Autodesk Inventor part; units mm, degrees
ref_plane "YZ Plane" through (0, 0, 0) normal (1, 0, 0) x (0, 1, 0)
ref_plane "XZ Plane" through (0, 0, 0) normal (0, 1, 0) x (-1, 0, 0)
ref_plane "XY Plane" through (0, 0, 0) normal (0, 0, 1) x (1, 0, 0)
sketch "Náčrt1" plane through (0, 0, 0) normal (0, 0, 1) x (1, 0, 0)
  line L0 (0, 0) -> (-28.2, 0)
  line L1 (-28.2, 0) -> (-28.2, -28.2)
  line L2 (-28.2, -28.2) -> (0, -28.2)
  line L3 (0, -28.2) -> (28.2, -28.2)
  line L4 (28.2, -28.2) -> (28.2, 28.2)
  line L5 (28.2, 28.2) -> (-28.2, 28.2)
  line L6 (-28.2, 28.2) -> (-28.2, 0)
  dimension "d0" = 28.2
  dimension "d1" = 28.2
  dimension "d2" = 28.2
  dimension "d3" = 56.4
extrude "Vysunutí1" add sketch "Náčrt1" along normal blind 54
sketch "Náčrt2" plane through (0, 0, 0) normal (0, 0, -1) x (-1, 0, 0)
  line L0 (28.2, 28.2) -> (28.2, -28.2)
  line L1 (-28.2, 28.2) -> (28.2, 28.2)
  line L2 (-28.2, -28.2) -> (-28.2, 28.2)
  line L3 (28.2, -28.2) -> (-28.2, -28.2)
  line L4 (28.2, 0) -> (28.2, -17.25)
  line L5 (17.25, -28.2) -> (-17.25, -28.2)
  line L6 (-17.25, -28.2) -> (-28.2, -17.25)
  line L7 (-28.2, -17.25) -> (-28.2, 17.25)
  line L8 (-28.2, 17.25) -> (-17.25, 28.2)
  line L9 (17.25, 28.2) -> (28.2, 17.25)
  line L10 (28.2, 17.25) -> (28.2, 0)
  line L11 (28.2, -28.2) -> (19.7, -28.2)
  line L12 (19.7, -28.2) -> (19.7, -19.7)
  line L13 (19.7, -19.7) -> (28.2, -19.7)
  line L14 (28.2, -19.7) -> (28.2, -28.2)
  line L15 (-28.2, -28.2) -> (-19.7, -28.2)
  line L16 (-19.7, -28.2) -> (-19.7, -19.7)
  line L17 (-19.7, -19.7) -> (-28.2, -19.7)
  line L18 (-28.2, -19.7) -> (-28.2, -28.2)
  line L19 (-28.2, 28.2) -> (-19.7, 28.2)
  line L20 (-19.7, 28.2) -> (-19.7, 19.7)
  line L21 (-19.7, 19.7) -> (-28.2, 19.7)
  line L22 (-28.2, 19.7) -> (-28.2, 28.2)
  line L23 (28.2, 28.2) -> (19.7, 28.2)
  line L24 (19.7, 28.2) -> (19.7, 19.7)
  line L25 (19.7, 19.7) -> (28.2, 19.7)
  line L26 (28.2, 19.7) -> (28.2, 28.2)
  line L27 (28.2, 17.25) -> (19.7, 19.7)
  line L28 (17.25, 28.2) -> (19.7, 19.7)
  line L29 (-17.25, 28.2) -> (-19.7, 19.7)
  line L30 (-28.2, 17.25) -> (-19.7, 19.7)
  line L31 (-28.2, -17.25) -> (-19.7, -19.7)
  line L32 (-19.7, -19.7) -> (-17.25, -28.2)
  line L33 (17.25, -28.2) -> (19.7, -19.7)
  line L34 (19.7, -19.7) -> (28.2, -17.25)
  line L35 (28.2, -17.25) -> (25.75, -19.7)
  line L36 (19.7, -25.75) -> (17.25, -28.2)
  point P0 (0, 0)
  dimension "d6" = 17.25
  dimension "d8" = 34.5
  dimension "d9" = 34.5
  dimension "d10" = 8.5
  dimension "d11" = 8.5
  dimension "d12" = 8.5
  dimension "d13" = 8.5
  dimension "d14" = 8.5
extrude "Vysunutí2" add sketch "Náčrt2" along normal blind 49 contours L0 L34 L33 L3 L32 L31 L2 L30 L29 L1 L28 L27
sketch "Náčrt3" plane through (0, 0, 54) normal (0, 0, 1) x (1, 0, 0)
  line L0 (-28.2, -28.2) -> (-28.2, 28.2)
  line L1 (28.2, -28.2) -> (-28.2, -28.2)
  line L2 (28.2, -28.2) -> (-28.2, -28.2)
  line L3 (-28.2, -28.2) -> (-28.2, 28.2)
  line L4 (-28.2, 28.2) -> (28.2, 28.2)
  line L5 (28.2, 28.2) -> (28.2, -28.2)
  point P0 (0, 0)
extrude "Vysunutí3" cut sketch "Náčrt3" against normal blind 49
fillet "Zaoblení1" radius 3 12 edges at (-17.25, -28.2, -24.5) (-19.7, -19.7, -24.5) (-28.2, -17.25, -24.5) (17.25, -28.2, -24.5) (19.7, -19.7, -24.5) (28.2, -17.25, -24.5) (28.2, 17.25, -24.5) (19.7, 19.7, -24.5) (17.25, 28.2, -24.5) (-17.25, 28.2, -24.5) (-19.7, 19.7, -24.5) (-28.2, 17.25, -24.5)
fillet "Zaoblení2" radius 4.6 4 edges at (28.2, 28.2, 2.5) (28.2, -28.2, 2.5) (-28.2, -28.2, 2.5) (-28.2, 28.2, 2.5)
sketch "Náčrt4" plane through (0, 0, 5) normal (0, 0, 1) x (1, 0, 0)
  circle A0 centre (0, 0) radius 19.05
  dimension "d21" = 38.1
extrude "Vysunutí4" add sketch "Náčrt4" along normal blind 1.6
sketch "Náčrt5" plane through (0, 0, 6.6) normal (0, 0, 1) x (1, 0, 0)
  circle A0 centre (0, 0) radius 19.05
  circle A1 centre (0, 0) radius 3.175
  dimension "d24" = 6.35
extrude "Vysunutí5" add sketch "Náčrt5" along normal blind 16 contours A1
sketch "Náčrt6" plane through (0, 0, 5) normal (0, 0, 1) x (1, 0, 0)
  arc A0 (-23.6, 28.2) -> (-28.2, 23.6) centre (-23.6, 23.6) ccw
hole "Díra1" at (-23.6, 23.6, 5) direction (0, 0, -1) diameter 5.2 end through all
sketch "Náčrt7" plane through (0, 0, 5) normal (0, 0, 1) x (1, 0, 0)
  arc A0 (28.2, 23.6) -> (23.6, 28.2) centre (23.6, 23.6) ccw
hole "Díra2" at (23.6, 23.6, 5) direction (0, 0, -1) diameter 5.2 end through all
sketch "Náčrt8" plane through (0, 0, 5) normal (0, 0, 1) x (1, 0, 0)
  arc A0 (23.6, -28.2) -> (28.2, -23.6) centre (23.6, -23.6) ccw
hole "Díra3" at (23.6, -23.6, 5) direction (0, 0, -1) diameter 5.2 end through all
sketch "Náčrt9" plane through (0, 0, 5) normal (0, 0, 1) x (1, 0, 0)
  arc A0 (-28.2, -23.6) -> (-23.6, -28.2) centre (-23.6, -23.6) ccw
hole "Díra4" at (-23.6, -23.6, 5) direction (0, 0, -1) diameter 5.2 end through all
sketch "Náčrt10" plane through (0, 0, -49) normal (0, 0, -1) x (-1, 0, 0)
  point P0 (0, 0)
hole "Díra5" at (0, 0, -49) direction (0, 0, 1) diameter 8.5 depth 5 countersink diameter 9 countersink angle 90
sketch "Náčrt15" plane through (0, 0, 22.6) normal (0, 0, 1) x (1, 0, 0)
  circle A0 centre (0, 0) radius 3.175
  line L0 (-1.9907, -2.4734) -> (-1.9907, 2.4734)
extrude "Vysunutí10" cut sketch "Náčrt15" against normal blind 10 contours L0 A0 picked at (-2.3855, 0)
chamfer "Zkosení1" distance 0.4 angle 45 3 edges at (-1.9907, 0, 22.6) (1.3712, -2.8637, 22.6) (1.3712, 2.8637, 22.6)
chamfer "Zkosení2" distance 0.5 angle 45 8 edges at (-23.6, 26.2, 5) (23.6, 26.2, 5) (23.6, -21, 5) (-23.6, -21, 5) (-23.6, -21, 0) (23.6, -21, 0) (23.6, 26.2, 0) (-23.6, 26.2, 0)
fillet "Zaoblení3" radius 0.8 24 edges at (0, 28.2, -49) (-16.7964, 27.5971, -49) (-18.5581, 23.6618, -49) (-20.0023, 20.0023, -49) (-23.6618, 18.5581, -49) (-27.5971, 16.7964, -49) (-28.2, 0, -49) (-27.5971, -16.7964, -49) (-23.6618, -18.5581, -49) (-20.0023, -20.0023, -49) (-18.5581, -23.6618, -49) (-16.7964, -27.5971, -49) (0, -28.2, -49) (16.7964, -27.5971, -49) (18.5581, -23.6618, -49) (20.0023, -20.0023, -49) (23.6618, -18.5581, -49) (27.5971, -16.7964, -49) (28.2, 0, -49) (27.5971, 16.7964, -49) (23.6618, 18.5581, -49) (20.0023, 20.0023, -49) (18.5581, 23.6618, -49) (16.7964, 27.5971, -49)
properties part number "nema 23 stepper" material "Steel, High Strength, Low Alloy"
Source: CAD feature listing. Evaluate the final solid. Frame: model axes, mm. A direction names the side the tool comes from. Round coordinates to 2 decimals unless told otherwise and drop trailing zeros. Loops run counter-clockwise (first coordinate to the right, second up) from the corner with the lowest first, then second, coordinate; pieces in that order, holes last. Notation, with made-up numbers: M -6.5,9.25 L 30.5,9.25 A19 cw 30.5,27.25 Z; hole C 65.5,-36 d2. An arc over 180 degrees is marked long. Use a Markdown table: item, result. Add a question column.
1. Mould query, pull axis X, two halves, no side actions, for faces 4 (the flat face through (-23, 20, 0)), 5 (the cylindrical face through (-18.348, 23.565, -48.759)), 6 (the cylindrical face through (26.14, 24.16, 2.47)). Classes: pulls with the +X half, pulls with the -X half, needs draft (parallel to the pull), parting line crosses it, or undercut.
2. Line query: line 1 (Y direction, x = -23.6, z = 1.35); line 2 (Y direction, x = -23, z = 3). Output: solid intervals per line, ascending.
3. Section query A-A on x = 0. Return the cut outline in (y, z) (3 decimals), then the cut area to 3 significant figures.
4. Section query B-B on y = 0. Return the cut outline in (x, z) (3 decimals), then the cut area to 3 significant figures.
5. Section query D-D on y = -10.5. Return the cut outline in (x, z).
6. Contact query for flat-ended pins moving along their axis: P1, Ø12, axis at x = -5, y = -2, coming from the +Z side; P2, Ø8.5, axis at x = -23.6, y = -23.6, coming from the -Z side; P3, Ø0.9, axis at x = -2.5, y = 0, coming from the +Z side; P4, Ø1.5, axis at y = 17, z = -10.5, coming from the +X side. Output: stop coordinate, or through.
7. Reachability of faces 1 (the flat face through (20, -23, 0)), 2 (the flat face through (-19.2, 0.4, 5)), 3 (the flat face through (18.55, 23.69, -23.76)) from +Z, -Z, +X, -X, +Y, -Y: full face, straight path, thin tool, end or side. Return the list, or none.
8. Section query C-C on z = -34.5. Return the cut outline in (x, y), then the cut area to 3 significant figures.
Reported:
| question | item | result |
|---|---|---|
| 1 | face 4 | needs draft |
| 1 | face 5 | pulls with the -X half |
| 1 | face 6 | undercut |
| 2 | line 1 | y = -28.2 to -26.2, -21 to 21, 26.2 to 28.2 |
| 2 | line 2 | y = -28.2 to -26.13, -21.07 to 21.07, 26.13 to 28.2 |
| 3 | outline | M -28.2,-48.2 A0.8 ccw -27.4,-49 L -4.5,-49 L -4.25,-48.75 L -4.25,-44 L 4.25,-44 L 4.25,-48.75 L 4.5,-49 L 27.4,-49 A0.8 ccw 28.2,-48.2 L 28.2,5 L 19.05,5 L 19.05,6.6 L 3.175,6.6 L 3.175,22.2 L 2.775,22.6 L -2.775,22.6 L -3.175,22.2 L -3.175,6.6 L -19.05,6.6 L -19.05,5 L -28.2,5 Z |
| 3 | area | 3,170 mm² |
| 4 | outline | M -28.2,-48.2 A0.8 ccw -27.4,-49 L -4.5,-49 L -4.25,-48.75 L -4.25,-44 L 4.25,-44 L 4.25,-48.75 L 4.5,-49 L 27.4,-49 A0.8 ccw 28.2,-48.2 L 28.2,5 L 19.05,5 L 19.05,6.6 L 3.175,6.6 L 3.175,22.2 L 2.775,22.6 L -1.591,22.6 L -1.991,22.2 L -1.991,12.6 L -3.175,12.6 L -3.175,6.6 L -19.05,6.6 L -19.05,5 L -28.2,5 Z |
| 4 | area | 3,150 mm² |
| 5 | outline | M -28.2,-48.2 A0.8 ccw -27.4,-49 L 27.4,-49 A0.8 ccw 28.2,-48.2 L 28.2,5 L 15.9,5 L 15.9,6.6 L -15.9,6.6 L -15.9,5 L -28.2,5 Z |
| 6 | P1 | stops at z = 22.6 |
| 6 | P2 | stops at z = 0 |
| 6 | P3 | stops at z = 12.6 |
| 6 | P4 | stops at x = 27.92 |
| 7 | face 1 | -Z, +X, -Y |
| 7 | face 2 | +Z |
| 7 | face 3 | -Z, +X, +Y |
| 8 | outline | M -28.2,-14.99 A3 ccw -26.03,-17.88 L -21.29,-19.24 A3 cw -19.24,-21.29 L -17.88,-26.03 A3 ccw -14.99,-28.2 L 14.99,-28.2 A3 ccw 17.88,-26.03 L 19.24,-21.29 A3 cw 21.29,-19.24 L 26.03,-17.88 A3 ccw 28.2,-14.99 L 28.2,14.99 A3 ccw 26.03,17.88 L 21.29,19.24 A3 cw 19.24,21.29 L 17.88,26.03 A3 ccw 14.99,28.2 L -14.99,28.2 A3 ccw -17.88,26.03 L -19.24,21.29 A3 cw -21.29,19.24 L -26.03,17.88 A3 ccw -28.2,14.99 Z |
| 8 | area | 2,800 mm² |
